The listing builds one solid part. Answer for the finished solid, in the listing's coordinates (mm). Face numbers are marked on the shaded views. Coordinates: 2 decimals unless noted, no trailing zeros. Order: outer loops, then holes, each group sorted by start corner. A loop starts at its lowest first (then second) coordinate and runs counter-clockwise, first axis right, second up. Notation, with made-up numbers: (50.25, 66) - (93.25, 66) arc R25 ccw to (93.25, 102) - close; hole circle Ø3 at (80.5, 58.5). An arc over 180 degrees is marked (long way). Use a Markdown table: item, result. Add a question column.
Item 1: Find the intervals of material crossed by line 1 along Z through (x, y) = (0, 12.55); line 2 along Z through (x, y) = (-0.5, 12.75); line 3 along Y through (x, z) = (-1, 0.5), in increasing order.
Item 2: The part is cut by section D-D, the plane y = 6.75. Give the vertices of the cut face in (x, z), then the cut area to 3 significant figures.
Item 3: The part is cut by section A-A, the plane z = 0. Give the vertices of the cut face in (x, y).
Item 4: The mould has two halves that part along Z. Classify the marked faces 1, 2, 3 and 4: released by +Z, released by -Z, zero draft, split by the parting line, or undercut.
Item 5: The part is cut by section B-B, the plane x = 0. Give the vertices of the cut face in (y, z), then the cut area to 3 significant figures.
Item 6: The part is cut by section C-C, the plane y = 9.25. Give the vertices of the cut face in (x, z), then the cut area to 3 significant figures.
Item 7: Flat-ended cylindrical pins translate along their axes: P1, Ø1.1, axis at x = -1, z = 0, coming from the -Y side; P2, Ø1.5, axis at x = 3, y = 12, coming from the -Z side; P3, Ø1.9, axis at x = 0.5, z = 0.5, coming from the +Y side. Find the tip coordinate at first contact, or state that the pin passes through.
Autodesk Inventor part; units mm, degrees
ref_plane "YZ Plane" through (0, 0, 0) normal (1, 0, 0) x (0, 1, 0)
ref_plane "XZ Plane" through (0, 0, 0) normal (0, 1, 0) x (-1, 0, 0)
ref_plane "XY Plane" through (0, 0, 0) normal (0, 0, 1) x (1, 0, 0)
sketch "Sketch1" plane through (0, 0, 0) normal (0, 1, 0) x (-1, 0, 0)
  circle A0 centre (0, 0) radius 4
  dimension "d0" = 8
extrude "Extrusion1" add sketch "Sketch1" along normal blind 14.68
sketch "Sketch2" plane through (0, 14.68, 0) normal (0, 1, 0) x (1, 0, 0)
  point P0 (0, 0)
sketch "Sketch3" plane through (0, 0, 0) normal (0, -1, 0) x (1, 0, 0)
  point P0 (0, 0)
hole "Hole1" at (0, 0, 0) direction (0, 1, 0) diameter 3.78 depth 6 countersink diameter 4.5 countersink angle 90
hole "Hole2" at (0, 14.68, 0) direction (0, -1, 0) diameter 3.78 depth 6 countersink diameter 4.5 countersink angle 90
properties part number "Button Spacer"
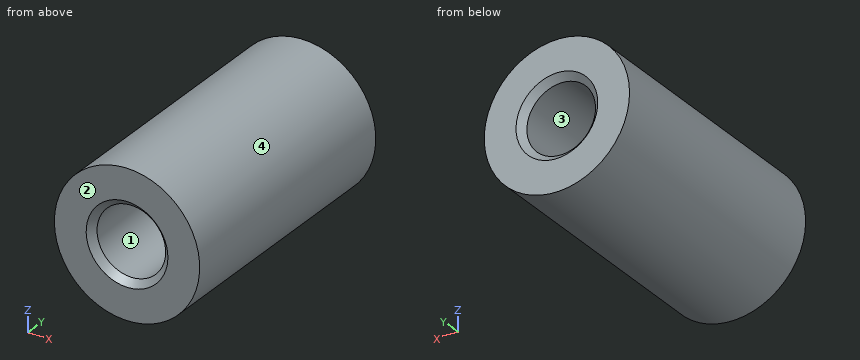
Solution:
| question | item | result |
|---|---|---|
| 1 | line 1 | z = -4 to -1.89, 1.89 to 4 |
| 1 | line 2 | z = -3.97 to -1.82, 1.82 to 3.97 |
| 1 | line 3 | y = 6 to 8.68 |
| 2 | outline | circle Ø8 at (0, 0) |
| 2 | area | 50.3 mm2 |
| 3 | outline | (-4, 0) - (-2.25, 0) - (-1.89, 0.36) - (-1.89, 6) - (1.89, 6) - (1.89, 0.36) - (2.25, 0) - (4, 0) - (4, 14.68) - (2.25, 14.68) - (1.89, 14.32) - (1.89, 8.68) - (-1.89, 8.68) - (-1.89, 14.32) - (-2.25, 14.68) - (-4, 14.68) - close |
| 4 | face 1 | undercut |
| 4 | face 2 | zero draft |
| 4 | face 3 | undercut |
| 4 | face 4 | split by the parting line |
| 5 | outline | (0, -4) - (14.68, -4) - (14.68, -2.25) - (14.32, -1.89) - (8.68, -1.89) - (8.68, 1.89) - (14.32, 1.89) - (14.68, 2.25) - (14.68, 4) - (0, 4) - (0, 2.25) - (0.36, 1.89) - (6, 1.89) - (6, -1.89) - (0.36, -1.89) - (0, -2.25) - close |
| 5 | area | 71.8 mm2 |
| 6 | outline | circle Ø8 at (0, 0); hole circle Ø3.78 at (0, 0) |
| 6 | area | 39.0 mm2 |
| 7 | P1 | stops at y = 6 |
| 7 | P2 | stops at z = -3.31 |
| 7 | P3 | stops at y = 8.68 |
